For this review, use the dimensioned drawing (mm, ordinates from the lowest corner) and the shaded views. A direction names the side the tool comes from. Round coordinates to 2 decimals unless told otherwise and drop trailing zeros. Loops run counter-clockwise (first coordinate to the right, second up) from the corner with the lowest first, then second, coordinate; pieces in that order, holes last. Notation, with made-up numbers: (31.5, 67.5) - (88.5, 67.5) arc R13 cw to (88.5, 88.5) - close; hole circle Ø9 at (45, 15.5). An arc over 180 degrees is marked (long way). Use one line per item in the form item = value. Start each with the question number.
(1) We need section A-A, the plane x = 20. Write out the cut boundary in (y, z), then the cut area to 3 significant figures.
(2) Machinability: for the marked faces 1 and 2, which of the approach directions +Z, -Z, +X, -X, +Y, -Y give a long, thin tool a straight path to every point of the face, cutting with its end or side? Answer none if there is none.
(3) We need section B-B, the plane y = 12.5. Write out the cut boundary in (x, z), then the cut area to 3 significant figures.
(4) For pin 1 (5 mm diameter, centred on x = 9.5, y = 20.5, fed in from +Z); pin 2 (5.5 mm diameter, centred on y = 14, z = 9, fed in from +X); pin 3 (7.5 mm diameter, centred on x = 20.5, z = 4.5, fed in from +Y), all flat-tipped, find the tip position at first contact; note any pin that passes through.
(5) We need section C-C, the plane z = 188.5. Write out the cut boundary in (x, y), then the cut area to 3 significant figures.
(6) We need section D-D, the plane x = 9. Write out the cut boundary in (y, z), then the cut area to 3 significant figures.
(7) Wall thickness on probe 1 along Z at (x, y) = (31, 10.25); probe 2 along X at (y, z) = (12.25, 189); probe 3 along Y at (x, z) = (20, 130): over which ranges is each line inside the solid? List them lowest first. Write a range as [from, to].
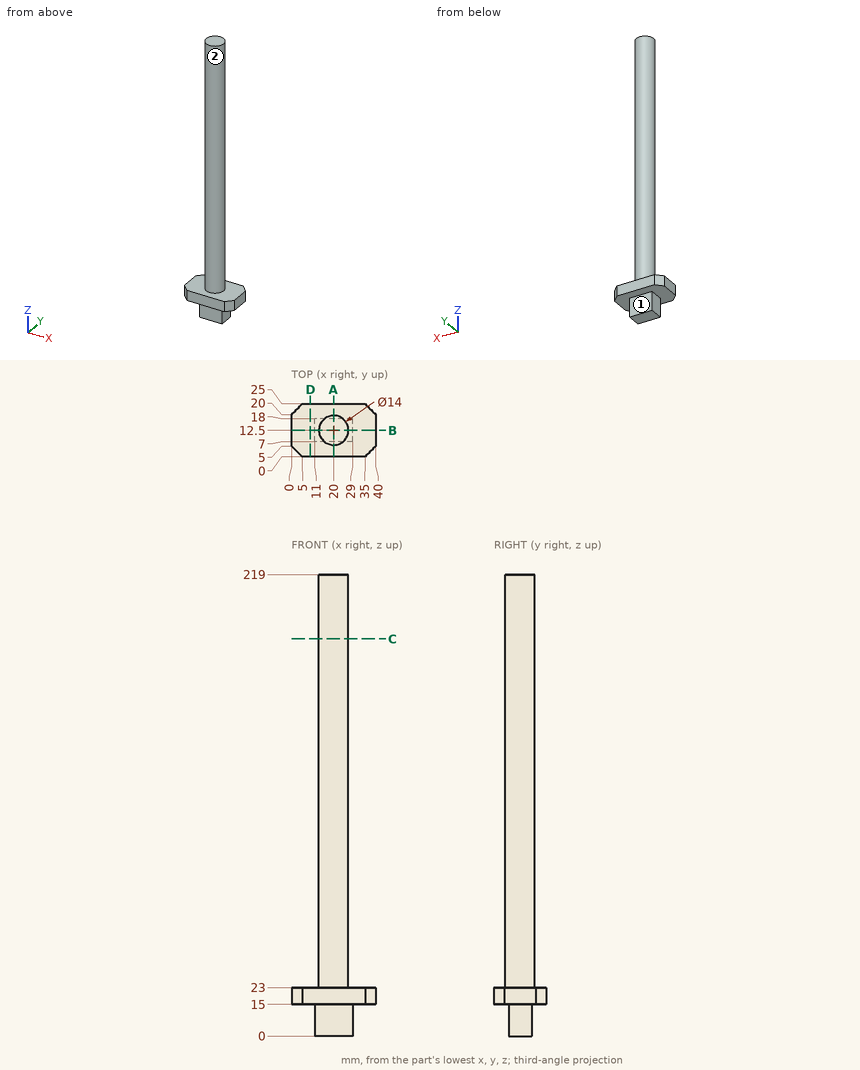
Data:
q1.outline = (0, 15) - (7, 15) - (7, 0) - (18, 0) - (18, 15) - (25, 15) - (25, 23) - (19.5, 23) - (19.5, 219) - (5.5, 219) - (5.5, 23) - (0, 23) - close
q1.area = 3,110 mm^2
q2.face_1 = -Z, +X, -X, +Y
q2.face_2 = +Z
q3.outline = (0, 15) - (11, 15) - (11, 0) - (29, 0) - (29, 15) - (40, 15) - (40, 23) - (27, 23) - (27, 219) - (13, 219) - (13, 23) - (0, 23) - close
q3.area = 3,330 mm^2
q4.pin_1 = 23
q4.pin_2 = 29
q4.pin_3 = 18
q5.outline = circle Ø14 at (20, 12.5)
q5.area = 154 mm^2
q6.outline = (0, 15) - (25, 15) - (25, 23) - (0, 23) - close
q6.area = 200 mm^2
q7.probe_1 = [15, 23]
q7.probe_2 = [13, 27]
q7.probe_3 = [5.5, 19.5]
